```python
from build123d import *

# Parameters (mm, degrees)
SKETCH1_W           = 66
SKETCH1_H           = 36
SKETCH1_R           = 4
SKETCH1_R_2         = 1.5
SKETCH1_W_2         = 7.7
SKETCH1_H_2         = 10
SKETCH1_W_3         = 22.5
SKETCH1_H_3         = 14
BOSS_EXTRUDE1_DEPTH = 2
SKETCH1_3_W         = 7.7
SKETCH1_3_H         = 10
BOSS_EXTRUDE2_DEPTH = 10
SKETCH1_4_W         = 22.5
SKETCH1_4_H         = 14
BOSS_EXTRUDE3_DEPTH = 7.5
SKETCH1_6_R         = 4
BOSS_EXTRUDE4_DEPTH = 10


with BuildPart() as part:
    # Sketch1 → Boss-Extrude1 (new body)
    # profile 1 of 6: a face of its own
    with BuildSketch(Plane.XY):
        with Locations((33, 18)):
            Rectangle(SKETCH1_W, SKETCH1_H)
        with Locations((13, 10)):
            Circle(SKETCH1_R, mode=Mode.SUBTRACT)
        with Locations((50, 10)):
            Circle(SKETCH1_R, mode=Mode.SUBTRACT)
        with Locations((2.5, 33.5)):
            Circle(SKETCH1_R_2, mode=Mode.SUBTRACT)
        with Locations((63.5, 33.5)):
            Circle(SKETCH1_R_2, mode=Mode.SUBTRACT)
        with Locations((2.5, 2.5)):
            Circle(SKETCH1_R_2, mode=Mode.SUBTRACT)
        with Locations((63.5, 2.5)):
            Circle(SKETCH1_R_2, mode=Mode.SUBTRACT)
        with Locations((61.15, 18)):
            Rectangle(SKETCH1_W_2, SKETCH1_H_2, mode=Mode.SUBTRACT)
        with Locations((34.75, 28)):
            Rectangle(SKETCH1_W_3, SKETCH1_H_3, mode=Mode.SUBTRACT)
        with Locations((4.85, 18)):
            Rectangle(SKETCH1_W_2, SKETCH1_H_2, mode=Mode.SUBTRACT)
    # profile 2 of 6: a face of its own
    with BuildSketch(Plane.XY):
        with Locations((61.15, 18)):
            Rectangle(SKETCH1_W_2, SKETCH1_H_2)
    # profile 3 of 6: a face of its own
    with BuildSketch(Plane.XY):
        with Locations((34.75, 28)):
            Rectangle(SKETCH1_W_3, SKETCH1_H_3)
    # profile 4 of 6: a face of its own
    with BuildSketch(Plane.XY):
        with Locations((50, 10)):
            Circle(SKETCH1_R)
    # profile 5 of 6: a face of its own
    with BuildSketch(Plane.XY):
        with Locations((13, 10)):
            Circle(SKETCH1_R)
    # profile 6 of 6: a face of its own
    with BuildSketch(Plane.XY):
        with Locations((4.85, 18)):
            Rectangle(SKETCH1_W_2, SKETCH1_H_2)
    extrude(amount=BOSS_EXTRUDE1_DEPTH)

    # Sketch1_3 → Boss-Extrude2 (add)
    with BuildSketch(Plane.XY):
        with Locations((4.85, 18)):
            Rectangle(SKETCH1_3_W, SKETCH1_3_H)
        with Locations((61.15, 18)):
            Rectangle(SKETCH1_3_W, SKETCH1_3_H)
    extrude(amount=-BOSS_EXTRUDE2_DEPTH)

    # Sketch1_4 → Boss-Extrude3 (add)
    with BuildSketch(Plane.XY):
        with Locations((34.75, 28)):
            Rectangle(SKETCH1_4_W, SKETCH1_4_H)
    extrude(amount=-BOSS_EXTRUDE3_DEPTH)

    # Sketch1_6 → Boss-Extrude4 (add)
    with BuildSketch(Plane.XY):
        with Locations((50, 10)):
            Circle(SKETCH1_6_R)
        with Locations((13, 10)):
            Circle(SKETCH1_6_R)
    extrude(amount=-BOSS_EXTRUDE4_DEPTH)


solid = part.part
```
Geometry check sheet. Reference: the model listing, model coordinates, mm. A direction names the side the tool comes from. Coordinates: 2 decimals unless noted, no trailing zeros. Write each loop counter-clockwise with the first axis right and the second up, starting at its lowest first coordinate (ties: lowest second). Pieces come first, ordered by that corner, then holes. Notation, with made-up numbers: (12.25, -38.75) -> (54.25, -38.75) arc R23 ccw to (54.25, -29.75) -> close; hole circle Ø11 at (36, 23.5). An arc over 180 degrees is marked (long way). Use CSV: the item, a comma, the result in double quotes. Start each with the question number.
Item 1: Mould release check, pull along X, two halves, no side actions. Record for faces 1 (the flat face through (33, 36, 1)), 2 (the flat face through (66, 18, 1)), 3 (the cylindrical face through (2.175, 32.036, 0.986)): released by +X, released by -X, zero draft, split by the parting line, or undercut.
Item 2: Set-up check for faces 4 (the flat face through (35, 35, -4)), 5 (the flat face through (61, 13, -5)), 6 (the flat face through (1, 18, -5)), 7 (the flat face through (61, 23, -5)), 8 (the flat face through (5, 13, -5)): record each of +Z, -Z, +X, -X, +Y, -Y from which the full face is reachable in a straight line by a thin tool's end or side.
Item 3: Cross-section at A-A, the plane x = 2.5. Record the cut outline in (y, z), plus the area to 3 significant figures.
Item 4: Thickness scan on line 1 (X direction, y = 22, z = -4.5); line 2 (Y direction, x = 63.5, z = 0.95); line 3 (X direction, y = 15, z = -3.75). Record the ranges inside material, lowest first.
Item 5: Cross-section at B-B, the plane y = 2.5. Record the cut outline in (x, z).
Item 6: Cross-section at D-D, the plane x = 43.5. Record the cut outline in (y, z), plus the area to 3 significant figures.
Item 7: Cross-section at C-C, the plane z = -3.5. Record the cut outline in (x, y).
Item 8: Depth check by flat-ended pin: pin 1 Ø3 at (y, z) = (16, -6) entering from +X; pin 2 Ø11 at (x, y) = (33.5, 30) entering from -Z; pin 3 Ø5 at (y, z) = (27, -5) entering from -X. Enter the tip coordinate at first touch or a pass-through.
Answers:
1,face 1,"zero draft"
1,face 2,"released by +X"
1,face 3,"undercut"
2,face 4,"-Z, +X, -X, +Y"
2,face 5,"-Z, +X, -Y"
2,face 6,"-Z, -X, +Y, -Y"
2,face 7,"-Z, +X, +Y"
2,face 8,"-Z, -X, -Y"
3,outline,"(0, 0) -> (1, 0) -> (1, 2) -> (0, 2) -> close; (4, 0) -> (13, 0) -> (13, -10) -> (23, -10) -> (23, 0) -> (32, 0) -> (32, 2) -> (4, 2) -> close; (35, 0) -> (36, 0) -> (36, 2) -> (35, 2) -> close"
3,area,"160 mm^2"
4,line 1,"1 to 8.7, 23.5 to 46, 57.3 to 65"
4,line 2,"0 to 1, 4 to 32, 35 to 36"
4,line 3,"1 to 8.7, 57.3 to 65"
5,outline,"(0, 0) -> (1, 0) -> (1, 2) -> (0, 2) -> close; (4, 0) -> (62, 0) -> (62, 2) -> (4, 2) -> close; (65, 0) -> (66, 0) -> (66, 2) -> (65, 2) -> close"
6,outline,"(0, 0) -> (21, 0) -> (21, -7.5) -> (35, -7.5) -> (35, 0) -> (36, 0) -> (36, 2) -> (0, 2) -> close"
6,area,"177 mm^2"
7,outline,"(1, 13) -> (8.7, 13) -> (8.7, 23) -> (1, 23) -> close; circle Ø8 at (13, 10); (23.5, 21) -> (46, 21) -> (46, 35) -> (23.5, 35) -> close; circle Ø8 at (50, 10); (57.3, 13) -> (65, 13) -> (65, 23) -> (57.3, 23) -> close"
8,pin 1,"x = 65"
8,pin 2,"z = -7.5"
8,pin 3,"x = 23.5"
